The model under review builds one solid part; all positions refer to its coordinate system, in mm. A direction names the side the tool comes from. Round coordinates to 2 decimals unless told otherwise and drop trailing zeros. Order: outer loops, then holes, each group sorted by start corner. A loop starts at its lowest first (then second) coordinate and runs counter-clockwise, first axis right, second up.
1) Machinability: for faces 1 (the face through (0.24, -0.02, 4.77)), 2 (the face through (4.76, 0.02, -4.77)), 3 (the face through (4.76, -0.02, 4.77)), which of the approach directions +Z, -Z, +X, -X, +Y, -Y give a long, thin tool a straight path to every point of the face, cutting with its end or side? Answer none if there is none.
2) Consider section B-B (x = 0.5). Give the boundary of the cut face in (y, z).
3) Mouldability with a two-part tool opening along Y and no side actions: class faces 4 (the face through (2.46, -1.5, 0.07)), 5 (the face through (2.476, 4.305, -2.543)), 6 (the face through (4.759, -4.123, -2.402)), 7 (the face through (5, 0, 2)) as pulls with the +Y half, pulls with the -Y half, needs draft (parallel to the pull), parting line crosses it, or undercut.
4) To check wall thickness, follow L1, parallel to Z at x = 3.15, y = 0; L2, parallel to Z at x = 4.75, y = 1.75; L3, parallel to Y at x = 2.85, z = 4. State the ranges of each line that lie inside material, in increasing order.
5) Consider section A-A (x = 3.4). Give the boundary of the cut face in (y, z), then the cut area to 3 significant figures.
6) Clearance check with flat-ended pins moving along their axes: P1, Ø3, axis at x = 2.5, z = -2, coming from the +Y side; P2, Ø1.5, axis at x = 1, y = 0.5, coming from the +Z side. State where each tip first meets the part, or that it passes through.
from build123d import *

# Parameters (mm, degrees)
F0_R     = 1.5
F1_DEPTH = 5
F2_R     = 0.8


with BuildPart() as f1:
    # F0 (on Right) → F1 (new body)
    with BuildSketch(Plane.YZ):
        Polygon((2.870718, -5.009223), (5.773473, -0.018497), (2.902755, 4.990726), (-2.870718, 5.009223), (-5.773473, 0.018497), (-2.902755, -4.990726), align=None)
        Circle(F0_R, mode=Mode.SUBTRACT)
    extrude(amount=F1_DEPTH)

    # F2
    f2_edges = [f1.edges().sort_by_distance(p)[0] for p in [
        (2.5, -2.870718, 5.009223),
        (2.5, 2.902755, 4.990726),
        (2.5, -5.773473, 0.018497),
        (2.5, -2.902755, -4.990726),
        (2.5, 2.870718, -5.009223),
        (2.5, 5.773473, -0.018497),
        (5, 4.338114, 2.486115),
        (0, 4.338114, 2.486115),
        (5, 4.322096, -2.51386),
        (0, 4.322096, -2.51386),
        (5, -0.016019, -4.999974),
        (0, -0.016019, -4.999974),
        (5, -4.338114, -2.486115),
        (0, -4.338114, -2.486115),
        (5, -4.322096, 2.51386),
        (0, -4.322096, 2.51386),
        (0, 0.016019, 4.999974),
        (5, 0.016019, 4.999974),
    ]]
    fillet(f2_edges, radius=F2_R)


solid = f1.part
Answer below:
1. face 1: +Z, -X, +Y
1. face 2: -Z, +X, -Y
1. face 3: +Z, +X, +Y
2. outline: (-5.49, -0.35) - (-3.08, -4.56) arc R0.74 ccw to (-2.44, -4.93) - (2.41, -4.95) arc R0.74 ccw to (3.05, -4.58) - (5.49, -0.39) arc R0.74 ccw to (5.49, 0.35) - (3.08, 4.56) arc R0.74 ccw to (2.44, 4.93) - (-2.41, 4.95) arc R0.74 ccw to (-3.05, 4.58) - (-5.49, 0.39) arc R0.74 ccw to start; hole circle Ø3 at (0, 0)
3. face 4: undercut
3. face 5: pulls with the +Y half
3. face 6: pulls with the -Y half
3. face 7: needs draft
4. L1: z = -5 to -1.5, 1.5 to 5
4. L2: z = -4.79 to 4.78
4. L3: y = -3.46 to 3.47
5. outline: (-5.54, -0.38) - (-3.13, -4.59) arc R0.8 ccw to (-2.44, -4.99) - (2.41, -5.01) arc R0.8 ccw to (3.1, -4.61) - (5.54, -0.42) arc R0.8 ccw to (5.54, 0.38) - (3.13, 4.59) arc R0.8 ccw to (2.44, 4.99) - (-2.41, 5.01) arc R0.8 ccw to (-3.1, 4.61) - (-5.54, 0.42) arc R0.8 ccw to start; hole circle Ø3 at (0, 0)
5. area: 79.3 mm2
6. P1: stops at y = 5.49
6. P2: stops at z = 5
